```python
from build123d import *

# Parameters (mm, degrees)
F0_W     = 30
F0_H     = 80
F1_DEPTH = 20
F2_R     = 3.5
F3_DEPTH = 20
F4_W     = 25
F4_H     = 10
F5_DEPTH = 20
F7_DEPTH = 20
F8_W     = 7.5
F8_H     = 20
F9_DEPTH = 20
F10_R    = 5
F11_R    = 5


with BuildPart() as f1:
    # F0 (on Top) → F1 (new body)
    with BuildSketch(Plane.XY):
        with Locations((15, 40)):
            Rectangle(F0_W, F0_H)
    extrude(amount=F1_DEPTH)

    # F2 (on Top) → F3 (cut)
    with BuildSketch(Plane.XY):
        with Locations((15, 15)):
            Circle(F2_R)
    extrude(amount=F3_DEPTH, mode=Mode.SUBTRACT)

    # F4 (on Top) → F5 (cut)
    with BuildSketch(Plane.XY):
        with Locations((15, 65)):
            Rectangle(F4_W, F4_H)
    extrude(amount=F5_DEPTH, mode=Mode.SUBTRACT)

    # F6 (on face) → F7 (cut)
    with BuildSketch(Plane(origin=(0, 80, 0), x_dir=(-1, 0, 0), z_dir=(0, 1, 0))):
        with BuildLine():
            ThreePointArc((-12, 10), (-15, 13), (-18, 10))
            Line((-18, 10), (-12, 10))
        make_face()
        with BuildLine():
            Line((-18, 20), (-18, 10))
            ThreePointArc((-18, 10), (-15, 13), (-12, 10))
            Line((-12, 10), (-12, 20))
            Line((-12, 20), (-18, 20))
        make_face()
        with BuildLine():
            Line((-12, 10), (-18, 10))
            ThreePointArc((-18, 10), (-15, 7), (-12, 10))
        make_face()
    extrude(amount=-F7_DEPTH, mode=Mode.SUBTRACT)

    # F8 (on face) → F9 (cut)
    with BuildSketch(Plane.XY.offset(20)):
        with Locations((26.25, 40)):
            Rectangle(F8_W, F8_H)
        with Locations((3.75, 40)):
            Rectangle(F8_W, F8_H)
    extrude(amount=-F9_DEPTH, mode=Mode.SUBTRACT)

    # F10
    f10_edges = [f1.edges().sort_by_distance(p)[0] for p in [
        (30, 30, 10),
        (0, 30, 10),
        (0, 0, 10),
        (30, 0, 10),
    ]]
    fillet(f10_edges, radius=F10_R)

    # F11
    f11_edges = [f1.edges().sort_by_distance(p)[0] for p in [
        (0, 80, 10),
        (0, 50, 10),
        (30, 50, 10),
        (30, 80, 10),
    ]]
    fillet(f11_edges, radius=F11_R)


solid = f1.part
```
Work out the finished part from the listing and answer in its coordinate system (mm). A direction names the side the tool comes from. Round coordinates to 2 decimals unless told otherwise and drop trailing zeros. Write each loop counter-clockwise with the first axis right and the second up, starting at its lowest first coordinate (ties: lowest second). Pieces come first, ordered by that corner, then holes.
1) A cutting plane is placed at A-A on x = 21.5. Determine the outline of the cut face in (y, z), and give its area (3 significant figures).
2) A cutting plane is placed at D-D on x = 15. Determine the outline of the cut face in (y, z).
3) Flat-ended cylindrical pins translate along their axes: P1, Ø1.5, axis at y = 35.5, z = 17.5, coming from the +X side; P2, Ø10, axis at y = 36, z = 3, coming from the -X side. Find the tip coordinate at first contact, or state that the pin passes through.
4) Determine the mould class of faces 4 (the face through (2, 51, 10)), 5 (the face through (28, 79, 10)), 6 (the face through (18, 75, 15)) for opening direction Y: pulls with the +Y half, pulls with the -Y half, needs draft (parallel to the pull), parting line crosses it, or undercut.
5) Consider probe 1 along Y at (x, z) = (15, 4.5); probe 2 along Y at (x, z) = (23.25, 12.25); probe 3 along Y at (x, z) = (15, 9.5). Determine where each line is inside the solid, lowest interval first.
6) A cutting plane is placed at C-C on y = 15. Determine the outline of the cut face in (x, z).
7) Which of the six approach directions +Z, -Z, +X, -X, +Y, -Y give full straight-line access (tool end or side, diameter ignored) to faces 1 (the face through (24, 50, 10)), 2 (the face through (6, 50, 10)), 3 (the face through (12, 70, 8))?
Entries:
1. outline: (0, 0) - (60, 0) - (60, 20) - (0, 20) - close; (70, 0) - (80, 0) - (80, 20) - (70, 20) - close
1. area: 1,400 mm2
2. outline: (0, 0) - (11.5, 0) - (11.5, 20) - (0, 20) - close; (18.5, 0) - (60, 0) - (60, 20) - (18.5, 20) - close; (70, 0) - (80, 0) - (80, 7) - (70, 7) - close
3. P1: stops at x = 22.5
3. P2: stops at x = 7.5
4. face 4: undercut
4. face 5: pulls with the +Y half
4. face 6: needs draft
5. probe 1: y = 0 to 11.5, 18.5 to 60, 70 to 80
5. probe 2: y = 0 to 30, 50 to 60, 70 to 80
5. probe 3: y = 0 to 11.5, 18.5 to 60
6. outline: (0, 0) - (11.5, 0) - (11.5, 20) - (0, 20) - close; (18.5, 0) - (30, 0) - (30, 20) - (18.5, 20) - close
7. face 1: +Z, -Z, +X
7. face 2: +Z, -Z, -X
7. face 3: +Z, -Z
